from build123d import *

# Parameters (mm, degrees)
ESBO_O6_R             = 0.8
CORTE_EXTRUS_O1_DEPTH = 35


with BuildPart() as part:
    # Esboço3 → Revolução1 (revolve)
    with BuildSketch(Plane.XY, mode=Mode.PRIVATE) as revolu_o1_sk:
        Polygon((0, 16), (0, 2), (-8, 2), (-8, 0), (-10, 0), (-10, 5), (-2, 5), (-2, 14), (-10, 14), (-10, 16), align=None)
    revolve(revolu_o1_sk.sketch.rotate(Axis((0, 0, 0), (-1, 0, 0)), 90), axis=Axis((0, 0, 0), (-1, 0, 0)))

    # Esboço6 → Corte-extrusão1 (cut, symmetric)
    with BuildSketch(Plane(origin=(0, 5, 0), x_dir=(1, 0, 0), z_dir=(0, 1, 0))):
        with Locations(Location((-5, 0, 0), (0, 0, 270))):
            Circle(ESBO_O6_R)
    extrude(amount=CORTE_EXTRUS_O1_DEPTH, both=True, mode=Mode.SUBTRACT)


solid = part.part
Can you work these out from the model? Positions are in its coordinate system, mm. A direction names the side the tool comes from. Give positions to 0.01 mm unless a question says otherwise; leave off trailing zeros. Loops run counter-clockwise (first coordinate to the right, second up) from the corner with the lowest first, then second, coordinate; pieces in that order, holes last. Notation, with made-up numbers: M -7.5,-9 L 33.5,-9 A18 ccw 33.5,-2 Z; hole C -35,19.25 d1. An arc over 180 degrees is marked long. One line per item, written item: value. Start each with the question number.
1) If we section it at D-D, the plane y = 0: Write out the boundary of the cut face in (x, z), and give its area (3 significant figures).
2) On a 3-axis mill with a long thin cutter (end or side, diameter ignored), from which of +Z, -Z, +X, -X, +Y, -Y can I reach the whole of each face in a straight line? I mean faces 1 (the face through (-8, 0, 0)), 2 (the face through (-5.78, 15, -0.17)), 3 (the face through (-2, 6, 0)). Say none if no direction works.
3) I'm going to push flat-ended pins straight in: pin 1 (2 mm diameter, centred on y = 0, z = 0, fed in from +X); pin 2 (1.5 mm diameter, centred on x = -1.5, y = 9, fed in from -Z); pin 3 (5 mm diameter, centred on x = -6, z = -4, fed in from -Y); pin 4 (1.3 mm diameter, centred on x = -5, z = 0, fed in from +Y). Where does each tip first touch, or does it pass through?
4) If we section it at B-B, the plane x = -9.5: Write out the boundary of the cut face in (y, z).
5) If we section it at A-A, the plane z = 0: Give the number of separate pieces and of enclosed holes in the cut face, and give its area (3 significant figures).
6) Thinking about a two-plate mould opening in Y: for faces 4 (the face through (-6.1, 12.4, -6.5)), 5 (the face through (-5.94, 4.88, 1.08)), 6 (the face through (-5.78, 3.44, -0.17)), 7 (the face through (-4.93, 15.62, 3.47)), which applies, +Y half, -Y half, draft (parallel to the pull), parting line (faces both ways), or undercut?
7) If we section it at C-C, the plane x = -5: Write out the boundary of the cut face in (y, z), and give its area (3 significant figures).
8) If I drill on line 1 (Y direction, x = -1.5, z = 0); line 2 (X direction, y = -14.45, z = 0); line 3 (Z direction, x = -5, y = 3.4), over which ranges is the centre line in solid material (lowest first)? Write a range as [from, to].
Completed:
1. outline: M -10,-16 L 0,-16 L 0,-2 L -8,-2 L -8,2 L 0,2 L 0,16 L -10,16 L -10,14 L -2,14 L -2,5 L -10,5 L -10,-5 L -2,-5 L -2,-14 L -10,-14 Z
1. area: 144 mm^2
2. face 1: +X
2. face 2: +Y, -Y
2. face 3: -X
3. pin 1: stops at x = -8
3. pin 2: stops at z = -13.71
3. pin 3: stops at y = -15.93
3. pin 4: passes through
4. outline: C 0,0 d32; C 0,0 d10; hole C 0,0 d28
5. separate pieces: 5
5. enclosed holes: 0
5. area: 128 mm^2
6. face 4: undercut
6. face 5: undercut
6. face 6: draft
6. face 7: parting line
7. outline: M -15.98,-0.8 A16 ccw 15.98,-0.8 L 13.98,-0.8 A14 cw -13.98,-0.8 Z; M -15.98,0.8 L -13.98,0.8 A14 cw 13.98,0.8 L 15.98,0.8 A16 ccw Z; M -4.94,-0.8 A5 ccw 4.94,-0.8 L 1.83,-0.8 A2 cw -1.83,-0.8 Z; M -4.94,0.8 L -1.83,0.8 A2 cw 1.83,0.8 L 4.94,0.8 A5 ccw Z
7. area: 238 mm^2
8. line 1: y = [-16, -2], [2, 16]
8. line 2: x = [-10, -5.8], [-4.2, 0]
8. line 3: z = [-15.63, -13.58], [-3.67, -0.8], [0.8, 3.67], [13.58, 15.63]
